Input: part model. Units: mm. Frame: model coordinates. A direction names the side the tool comes from. Give positions to 0.01 mm unless a question says otherwise; leave off trailing zeros. Loops run counter-clockwise (first coordinate to the right, second up) from the corner with the lowest first, then second, coordinate; pieces in that order, holes last.
Autodesk Inventor part; units mm, degrees
ref_plane "Work Plane1" through (-0.4, 0, 0) normal (1, 0, 0) x (0, 0, -1)
ref_plane "YZ Plane" through (0, 0, 0) normal (1, 0, 0) x (0, 1, 0)
ref_plane "XZ Plane" through (0, 0, 0) normal (0, 1, 0) x (-1, 0, 0)
sketch "Sketch1" plane through (0, 0, 0) normal (1, 0, 0) x (0, 1, 0)
  circle A0 centre (0, 0) radius 2.525
  circle A1 centre (0, 0) radius 7.85
  dimension "d0" = 5.05
  dimension "d1" = 15.7
extrude "Extrusion1" add sketch "Sketch1" against normal blind 11
sketch "Sketch2" plane through (0, 0, 0) normal (1, 0, 0) x (0, 0, -1)
  circle A0 centre (0, 0) radius 4.5
  circle A1 centre (0, 0) radius 6.75
  dimension "d4" = 9
  dimension "d5" = 13.5
extrude "Extrusion2" cut sketch "Sketch2" against normal blind 0.1
sketch "Sketch3" plane through (-11, 0, 0) normal (-1, 0, 0) x (0, 0, 1)
  circle A0 centre (0, 0) radius 6.75
  circle A1 centre (0, 0) radius 4.5
extrude "Extrusion3" cut sketch "Sketch3" against normal blind 0.1
ref_plane "Work Plane1" through (-0.4, 0, 0) normal (1, 0, 0) x (0, 0, -1)
sketch "Sketch4" plane through (-0.4, 0, 0) normal (1, 0, 0) x (0, 0, -1)
  circle A0 centre (0, 0) radius 7.85
  circle A1 centre (0, 0) radius 12
  dimension "d11" = 24
extrude "Extrusion4" add sketch "Sketch4" against normal blind 10.2
chamfer "Chamfer1" distance 2.1 angle 45 1 edges at (-0.4, 0, 12) measured on face at (-0.4, -1.2727, -10.4814)
chamfer "Chamfer2" distance 2.1 angle 45 1 edges at (-10.6, 0, 12) measured on face at (-10.6, -1.2727, -10.4814)
properties part number "M5 V Wheel"
(1) Ray query, probe 1 along X at (y, z) = (-2.5, -7.5); probe 2 along Z at (x, y) = (-0.5, 0.5) (1 decimal); probe 3 along Z at (x, y) = (-7.5, -0.75). Return the intervals inside material, ascending.
Values follow:
probe 1: x = -10.6 to -0.4
probe 2: z = -10 to -2.5, 2.5 to 10
probe 3: z = -11.98 to -2.41, 2.41 to 11.98
(2) Pin query (flat end, axial travel): pin 1 Ø1 at (y, z) = (4.5, 3.5) entering from +X; pin 2 Ø12 at (y, z) = (0, 0) entering from +X; pin 3 Ø1 at (x, y) = (-6.5, 1.5) entering from -Z; pin 4 Ø1.5 at (x, z) = (-4, 2.5) entering from +Y. Return the tip coordinate at first contact, or that it passes through.
Values follow:
pin 1: stops at x = -0.1
pin 2: stops at x = 0
pin 3: stops at z = -11.96
pin 4: stops at y = 11.87
(3) Cut plane B-B (x = -6). Return the cut outline in (y, z) (3 decimals).
Values follow:
outline: circle Ø24 at (0, 0); hole circle Ø5.05 at (0, 0)
(4) Mould query, pull axis Z, two halves, no side actions, for faces 1 (the flat face through (0, -4, 6)), 2 (the cylindrical face through (-5.42, 2.41, 0.76)), 3 (the conical face through (-10.47, 0.44, 10.02)). Classes: +Z half, -Z half, draft (parallel to the pull), parting line (faces both ways), or undercut.
Values follow:
face 1: draft
face 2: undercut
face 3: parting line
(5) Cut plane A-A (x = -1.5). Return the cut outline in (y, z) (3 decimals).
Values follow:
outline: circle Ø22 at (0, 0); hole circle Ø5.05 at (0, 0)
(6) Reachability of faces 4 (the flat face through (-11, 2, -2)), 5 (the flat face through (-10.6, 4, 7)), 6 (the flat face through (-0.4, 4, 7)) from +Z, -Z, +X, -X, +Y, -Y: full face, straight path, thin tool, end or side. Return the list, or none.
Values follow:
face 4: +Z, -Z, -X, +Y, -Y
face 5: -X
face 6: +X
